Read the model definition and answer for the solid it produces. Units are mm, in the model's axes. A direction names the side the tool comes from. Round coordinates to 2 decimals unless told otherwise and drop trailing zeros. Order: outer loops, then holes, each group sorted by start corner. A loop starts at its lowest first (then second) coordinate and runs counter-clockwise, first axis right, second up. Notation, with made-up numbers: M -3,87.25 L 46,87.25 A28 cw 46,108.25 Z; hole C 57.25,13.5 d11. An arc over 180 degrees is marked long. Answer as CSV lines item,"result".
Autodesk Inventor part; units mm, degrees
ref_plane "YZ Plane" through (0, 0, 0) normal (1, 0, 0) x (0, 1, 0)
ref_plane "XZ Plane" through (0, 0, 0) normal (0, 1, 0) x (-1, 0, 0)
ref_plane "XY Plane" through (0, 0, 0) normal (0, 0, 1) x (1, 0, 0)
sketch "Sketch1" plane through (0, 0, 0) normal (0, 0, 1) x (1, 0, 0)
  circle A0 centre (0, 0) radius 4.75
  circle A1 centre (0, 0) radius 9
  line L0 (-18, 9) -> (-18, -49.1769)
  line L1 (-18, 9) -> (10.681, 9)
  line L2 (4.1136, -2.375) -> (10.681, 9)
  line L3 (-0.2887, 9) -> (-4.1136, 2.375)
  line L4 (10.681, 9) -> (15.5885, 9)
  line L5 (4.1136, -2.375) -> (7.7942, -4.5) construction
  line L6 (7.7942, -4.5) -> (15.5885, 9)
  line L7 (7.7942, -4.5) -> (-18, -49.1769)
  line L8 (-18, -31) -> (-7.5056, -31)
  line L9 (-13, 9) -> (-13, -31)
  dimension "d1" = 18
  dimension "d0" = 9.5
  dimension "d2" = 18
  dimension "d5" = 120
  dimension "d7" = 60
  dimension "d8" = 40
  dimension "d9" = 5
extrude "Extrusion1" add sketch "Sketch1" along normal blind 6 contours A0 L2 A1 L3 | A1 L7 L8 L9 L1 L3 | L2 L4 L6 A1 | L9 L8 L0 L1 picked at (-2.2884, 6.6758)
extrude "Extrusion2" add sketch "Sketch1" along normal blind 20 contours L9 L8 L0 L1
sketch "Sketch2" plane through (-18, -31, 0) normal (-1, 0, 0) x (0, 0, 1)
  line L0 (0, 40) -> (0, 0)
  line L1 (0, 0) -> (20, 0)
  line L2 (20, 40) -> (20, 0)
  line L3 (0, 40) -> (20, 40)
  circle A0 centre (10, 30) radius 1.6
  circle A1 centre (10, 10) radius 1.6
  point P0 (0, 31)
  dimension "d14" = 3.2
  dimension "d15" = 3.2
  dimension "d16" = 10
  dimension "d17" = 10
  dimension "d18" = 10
extrude "Extrusion3" cut sketch "Sketch2" against normal blind 6 contours A0 | A1
fillet "Fillet1" radius 1 3 edges at (15.5885, 9, 3) (10.681, 9, 3) (-0.2887, 9, 3)
fillet "Fillet2" radius 5 3 edges at (-7.5056, -31, 3) (-15.5, -31, 20) (-15.5, 9, 20)
chamfer "Chamfer1" distance 1 angle 45 1 edges at (-13, -11, 6)
properties part number "wheel holder"
Item 1: A cutting plane is placed at D-D, the plane y = -21. Determine the outline of the cut face in (x, z).
Ans:
outline,"M -18,0 L -1.73,0 L -1.73,6 L -12,6 L -13,7 L -13,8.4 L -18,8.4 Z; M -18,11.6 L -13,11.6 L -13,20 L -18,20 Z"
Item 2: A cutting plane is placed at A-A, the plane z = 10. Determine the outline of the cut face in (x, y).
Ans:
outline,"M -18,-31 L -13,-31 L -13,-22.6 L -18,-22.6 Z; M -18,-19.4 L -13,-19.4 L -13,-2.6 L -18,-2.6 Z; M -18,0.6 L -13,0.6 L -13,9 L -18,9 Z"
Item 3: A cutting plane is placed at B-B, the plane y = -1. Determine the outline of the cut face in (x, z), and give its area (3 significant figures).
Ans:
outline,"M -18,0 L -4.64,0 L -4.64,6 L -12,6 L -13,7 L -13,8.4 L -18,8.4 Z; M -18,11.6 L -13,11.6 L -13,20 L -18,20 Z; M 4.91,0 L 9.81,0 L 9.81,6 L 4.91,6 Z"
area,"164 mm2"
Item 4: Determine the mould class of faces 1 (the face through (-7.924, -30.348, 3.042)), 2 (the face through (-15, 8, 18)), 3 (the face through (-2.6, 5, 3)) for opening direction Y: +Y half, -Y half, draft (parallel to the pull), parting line (faces both ways), or undercut.
Ans:
face 1,"-Y half"
face 2,"+Y half"
face 3,"undercut"
Item 5: A tool of negligible diameter and unlimited length cuts with its end or side. For faces 4 (the face through (7.21, 2.99, 2.96)), 5 (the face through (-13, -11, 13)), 6 (the face through (-1.15, 8.49, 3.04)), from which of +Z, -Z, +X, -X, +Y, -Y can it reach the whole face along a straight path? Write none if from no direction.
Ans:
face 4,"+Z, -Z, +Y"
face 5,"+Z, +X, +Y, -Y"
face 6,"+Z, -Z"
Item 6: Find the intervals of material crossed by probe 1 along Y at (x, z) = (-16.05, 10); probe 2 along X at (y, z) = (-21, 11.75); probe 3 along Z at (x, y) = (13, 7.5), in increasing order. Write a range as [from, to].
Ans:
probe 1,"[-31, -22.6], [-19.4, -2.6], [0.6, 9]"
probe 2,"[-18, -13]"
probe 3,"[0, 6]"
Item 7: A cutting plane is placed at C-C, the plane z = 2. Determine the outline of the cut face in (x, y) (3 decimals).
Ans:
outline,"M -18,-31 L -10.392,-31 A5 ccw -6.062,-28.5 L 7.794,-4.5 L 14.722,7.5 A1 ccw 13.856,9 L 11.258,9 A1 ccw 10.392,8.5 L 4.114,-2.375 A4.75 cw -4.114,2.375 L -1.155,7.5 A1 ccw -2.021,9 L -18,9 Z"
Item 8: Flat-ended cylindrical pins translate along their axes: pin 1 (3 mm diameter, centred on x = -5, y = 1.5, fed in from +Z); pin 2 (2 mm diameter, centred on y = -8.5, z = 11, fed in from +X); pin 3 (1 mm diameter, centred on y = -7.5, z = 7, fed in from +X). Find the tip coordinate at first contact, or state that the pin passes through.
Ans:
pin 1,"z = 6"
pin 2,"x = -13"
pin 3,"x = -12.5"
